from build123d import *

# Parameters (mm, degrees)
SKETCH003_W  = 73
SKETCH003_H  = 0.6
PAD003_DEPTH = 49.5
SKETCH004_W  = 1
SKETCH004_H  = 49.5
PAD004_DEPTH = 2
FILLET005_R  = 0.4
FILLET006_R  = 0.2


with BuildPart() as part:
    # Sketch003 → Pad003 (new body)
    with BuildSketch(Plane.XY):
        Rectangle(SKETCH003_W, SKETCH003_H)
    extrude(amount=PAD003_DEPTH)

    # Sketch004 (on Face3 of Pad003) → Pad004 (join)
    with BuildSketch(Plane.XZ.offset(0.3)):
        with Locations((-1.25, 24.75)):
            Rectangle(SKETCH004_W, SKETCH004_H)
        with Locations((1.25, 24.75)):
            Rectangle(SKETCH004_W, SKETCH004_H)
    extrude(amount=PAD004_DEPTH)

    # Fillet005
    fillet005_edges = [part.edges().sort_by_distance(p)[0] for p in [
        (-1.75, -2.3, 24.75),
        (-0.75, -2.3, 24.75),
        (0.75, -2.3, 24.75),
        (1.75, -2.3, 24.75),
    ]]
    fillet(fillet005_edges, radius=FILLET005_R)

    # Fillet006
    fillet006_edges = [part.edges().sort_by_distance(p)[0] for p in [
        (-36.5, -0.3, 24.75),
        (-36.5, 0.3, 24.75),
        (36.5, -0.3, 24.75),
        (36.5, 0.3, 24.75),
    ]]
    fillet(fillet006_edges, radius=FILLET006_R)


with BuildPart() as part_1:
    # Body002 placement: moved
    add(part.part.moved(Location((0, -44, -241))))


solid = part_1.part
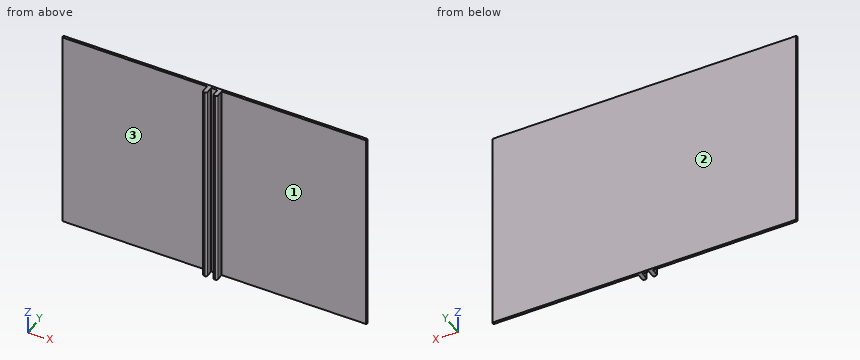
For this review, take the finished solid that the model builds, in its own axes (mm). Face numbers are marked on the shaded views. A direction names the side the tool comes from. Round coordinates to 2 decimals unless told otherwise and drop trailing zeros. Order: outer loops, then holes, each group sorted by start corner. A loop starts at its lowest first (then second) coordinate and runs counter-clockwise, first axis right, second up. Notation, with made-up numbers: (13.5, 3.25) -> (24.5, 3.25) arc R21 cw to (24.5, 31.25) -> close; hole circle Ø8 at (45.25, -30). An arc over 180 degrees is marked (long way). Put each result on its own line as item: value.
Q1. For probe 1 along X at (y, z) = (-45.8, -221); probe 2 along Y at (x, z) = (-19, -231.5), list the stretches that pass through material, from the lowest coordinate up. Write a range as [from, to].
Check result:
probe 1: [-1.75, -0.75], [0.75, 1.75]
probe 2: [-44.3, -43.7]
Q2. Add section C-C on x = -20.5. Write out the cut boundary in (y, z), plus the area to 3 significant figures.
Check result:
outline: (-44.3, -241) -> (-43.7, -241) -> (-43.7, -191.5) -> (-44.3, -191.5) -> close
area: 29.7 mm2
Q3. Insertion check: pin 1 Ø1.3 at (y, z) = (-45, -204.5) entering from +X; pin 2 Ø5 at (x, z) = (6.5, -231.5) entering from -Y; pin 3 Ø0.5 at (y, z) = (-45.5, -212) entering from -X. Each pin has a flat end and moves straight along its axis. Give the tip position at first contact, or say it passes through.
Check result:
pin 1: x = 1.75
pin 2: y = -44.3
pin 3: x = -1.75
Q4. Add section B-B on z = -228. Write out the cut boundary in (x, y), plus the area to 3 significant figures.
Check result:
outline: (-36.5, -44.1) arc R0.2 ccw to (-36.3, -44.3) -> (-1.75, -44.3) -> (-1.75, -45.9) arc R0.4 ccw to (-1.35, -46.3) -> (-1.15, -46.3) arc R0.4 ccw to (-0.75, -45.9) -> (-0.75, -44.3) -> (0.75, -44.3) -> (0.75, -45.9) arc R0.4 ccw to (1.15, -46.3) -> (1.35, -46.3) arc R0.4 ccw to (1.75, -45.9) -> (1.75, -44.3) -> (36.3, -44.3) arc R0.2 ccw to (36.5, -44.1) -> (36.5, -43.9) arc R0.2 ccw to (36.3, -43.7) -> (-36.3, -43.7) arc R0.2 ccw to (-36.5, -43.9) -> close
area: 47.6 mm2
Q5. Machinability: for the marked faces 1, 2 and 3, which of the approach directions +Z, -Z, +X, -X, +Y, -Y give a long, thin tool a straight path to every point of the face, cutting with its end or side? Answer none if there is none.
Check result:
face 1: +Z, -Z, +X, -Y
face 2: +Z, -Z, +X, -X, +Y
face 3: +Z, -Z, -X, -Y
Q6. Add section A-A on y = -44.7. Write out the cut boundary in (x, z), plus the area to 3 significant figures.
Check result:
outline: (-1.75, -241) -> (-0.75, -241) -> (-0.75, -191.5) -> (-1.75, -191.5) -> close; (0.75, -241) -> (1.75, -241) -> (1.75, -191.5) -> (0.75, -191.5) -> close
area: 99.0 mm2
